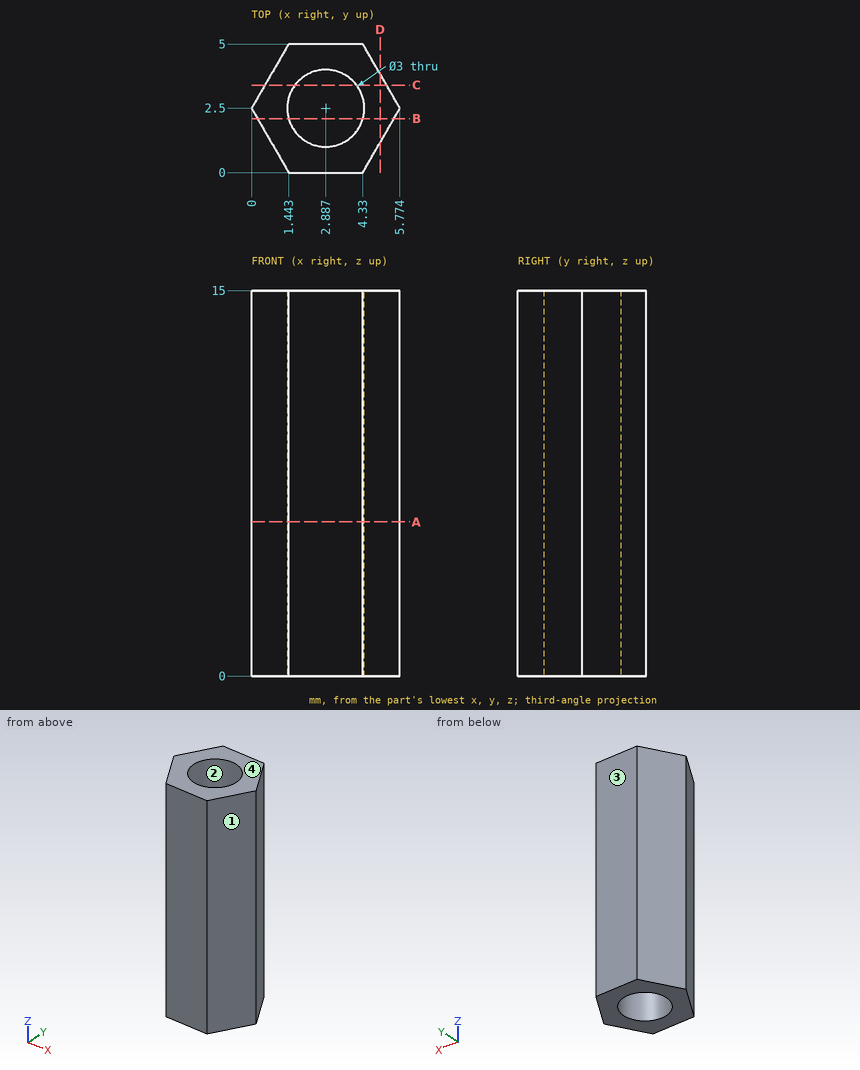
Geometry check sheet. Reference: drawing and pictorial views, mm from the part's lowest x, y, z. Round coordinates to 2 decimals unless told otherwise and drop trailing zeros. Loops run counter-clockwise (first coordinate to the right, second up) from the corner with the lowest first, then second, coordinate; pieces in that order, holes last. Notation, with made-up numbers: M 86.5,39.25 L 134.5,39.25 A25 ccw 134.5,67.25 Z; hole C -10.5,-34 d8. An arc over 180 degrees is marked long. Return JSON: item names as keys, results as strings. Group by question number.
(1) Section check D-D, the plane x = 5. Enter the section's corners in (y, z), and give its area (3 significant figures).
(2) Scan lines: line 1 along Y through (x, z) = (2.85, 3.5); line 2 along X through (y, z) = (2.15, 1) (1 decimal); line 3 along X through (y, z) = (3.85, 5.5) (1 decimal). Record each from-to range of solid material in increasing order. Write a range as [from, to].
(3) Section check C-C, the plane y = 3.4. Enter the section's corners in (x, z).
(4) Mould release check, pull along Y, two halves, no side actions. Record for the marked faces 1, 2, 3 and 4: pulls with the +Y half, pulls with the -Y half, needs draft (parallel to the pull), parting line crosses it, or undercut.
(5) Section check A-A, the plane z = 6. Enter the section's corners in (x, y).
(6) Go/stop test with flat-tipped pins: pin 1 (2.5 mm diameter, centred on x = 2.89, y = 2.5, fed in from +Z); pin 2 (1.5 mm diameter, centred on y = 1, z = 13, fed in from -X). Record where each tip stops, or that it passes through.
(7) Section check B-B, the plane y = 2.1. Enter the section's corners in (x, z).
Data:
{
 "1": {"outline": "M 1.16,0 L 3.84,0 L 3.84,15 L 1.16,15 Z", "area": "40.2 mm²"},
 "2": {"line 1": "[0, 1], [4, 5]", "line 2": "[0.2, 1.4], [4.3, 5.6]", "line 3": "[0.8, 2.2], [3.5, 5]"},
 "3": {"outline": "M 0.52,0 L 1.69,0 L 1.69,15 L 0.52,15 Z; M 4.09,0 L 5.25,0 L 5.25,15 L 4.09,15 Z"},
 "4": {"face 1": "pulls with the -Y half", "face 2": "undercut", "face 3": "pulls with the +Y half", "face 4": "needs draft"},
 "5": {"outline": "M 0,2.5 L 1.44,0 L 4.33,0 L 5.77,2.5 L 4.33,5 L 1.44,5 Z; hole C 2.89,2.5 d3"},
 "6": {"pin 1": "through", "pin 2": "x = 0.43"},
 "7": {"outline": "M 0.23,0 L 1.44,0 L 1.44,15 L 0.23,15 Z; M 4.33,0 L 5.54,0 L 5.54,15 L 4.33,15 Z"}
}
